Here's how the part is built. I have some questions about the finished solid (model axes, mm). Face numbers are marked on the shaded views. A direction names the side the tool comes from. Round coordinates to 2 decimals unless told otherwise and drop trailing zeros. Loops run counter-clockwise (first coordinate to the right, second up) from the corner with the lowest first, then second, coordinate; pieces in that order, holes last. Notation, with made-up numbers: (44.25, -12.5) -> (58.25, -12.5) arc R18 cw to (58.25, 17.5) -> close; hole circle Ø3 at (21, 34.25). An arc over 180 degrees is marked (long way). One line per item, written item: value. Start each with the question number.
```python
from build123d import *

# Parameters (mm, degrees)
SKETCH_1_R              = 1.75
EXTRUDE_1_DEPTH         = 3.5
EXTRUDE_2_DEPTH         = 1.5
EXTRUDE_2_DEPTH_BACK    = 13.5
SKETCH_2_R              = 5
SKETCH_2_R_2            = 4
CUT_EXTRUDE_START       = -3.5
CUT_EXTRUDE_1_OUTLINE_R = 4
CUT_EXTRUDE_1_DEPTH     = 3.5


# Read off the part's stored shape, not the designer's step: the extrude step
with BuildPart() as part:
    # Sketch 1 → Extrude 1 (new body)
    with BuildSketch(Plane.XY):
        with BuildLine():
            Line((-9.5, -5.5), (9.5, -5.5))
            ThreePointArc((9.5, -5.5), (11, 0), (9.5, 5.5))
            Line((9.5, 5.5), (-9.5, 5.5))
            ThreePointArc((-9.5, 5.5), (-11, 0), (-9.5, -5.5))
        make_face()
        with Locations((8, 0)):
            Circle(SKETCH_1_R, mode=Mode.SUBTRACT)
        with Locations((-8, 0)):
            Circle(SKETCH_1_R, mode=Mode.SUBTRACT)
    extrude(amount=EXTRUDE_1_DEPTH)

    # Sketch 2 → Extrude 2 (add, two sides: drawn at the far end of the back side and taken through both)
    with BuildSketch(Plane(origin=(0, 0, 0), x_dir=(-1, 0, 0), z_dir=(0, 0, -1)).offset(-EXTRUDE_2_DEPTH_BACK)):
        Circle(SKETCH_2_R)
        Circle(SKETCH_2_R_2, mode=Mode.SUBTRACT)
    extrude(amount=EXTRUDE_2_DEPTH + EXTRUDE_2_DEPTH_BACK)

    # Cut-Extrude 1 outline → Cut-Extrude 1 (cut)
    with BuildSketch(Plane(origin=(0, 0, 0), x_dir=(-1, 0, 0), z_dir=(0, 0, -1)).offset(CUT_EXTRUDE_START)):
        Circle(CUT_EXTRUDE_1_OUTLINE_R)
    extrude(amount=CUT_EXTRUDE_1_DEPTH, mode=Mode.SUBTRACT)


solid = part.part
```
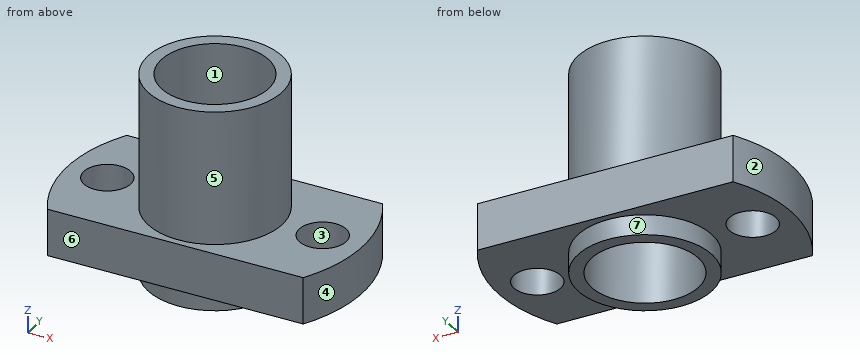
Q1. Which directions (+Z, -Z, +X, -X, +Y, -Y) give clear straight access to the entire face, cutting with the end or side of a thin tool? Please do the marked faces 5, 6 and 7.
Q2. I want a section at B-B on x = -8. Please give me the cut outline in (y, z).
Q3. If we mould it in two halves opening along X, with no side actions, what happens to the marked faces 1, 2, 3 and 4? For each: released by +X, released by -X, zero draft, split by the parting line, or undercut.
Q4. I want a section at A-A on y = 0. Please give me the cut outline in (x, z).
Q5. I want a section at D-D on y = -4.25. Please give me the cut outline in (x, z), plus the area to 3 significant figures.
Q6. Will these pins go through, and if not, where does the flat tip stop? P1, Ø2, axis at y = -3.5, z = 8.5, coming from the +X side; P2, Ø3.5, axis at x = -1.5, y = 2, coming from the -Z side; P3, Ø4, axis at y = -1.5, z = 6, coming from the +X side; P4, Ø2, axis at x = -1, z = 11.5, coming from the -Y side.
Q7. I want a section at C-C on z = 2.75. Please give me the cut outline in (x, y), plus the area to 3 significant figures.
Q8. If I drill on line 1 along Y through (x, z) = (8, 1); line 2 along X through (y, z) = (0.75, 3.25); line 3 along Y through (x, z) = (0, 9), over which ranges is the centre line in solid material (lowest first)?
Answers below:
1. face 5: +Z
1. face 6: +Z, -Z, +X, -X, -Y
1. face 7: -Z
2. outline: (-5.5, 0) -> (-1.75, 0) -> (-1.75, 3.5) -> (-5.5, 3.5) -> close; (1.75, 0) -> (5.5, 0) -> (5.5, 3.5) -> (1.75, 3.5) -> close
3. face 1: undercut
3. face 2: released by -X
3. face 3: undercut
3. face 4: released by +X
4. outline: (-11, 0) -> (-9.75, 0) -> (-9.75, 3.5) -> (-11, 3.5) -> close; (-6.25, 0) -> (-5, 0) -> (-5, -1.5) -> (-4, -1.5) -> (-4, 13.5) -> (-5, 13.5) -> (-5, 3.5) -> (-6.25, 3.5) -> close; (4, -1.5) -> (5, -1.5) -> (5, 0) -> (6.25, 0) -> (6.25, 3.5) -> (5, 3.5) -> (5, 13.5) -> (4, 13.5) -> close; (9.75, 0) -> (11, 0) -> (11, 3.5) -> (9.75, 3.5) -> close
5. outline: (-10.13, 0) -> (-2.63, 0) -> (-2.63, -1.5) -> (2.63, -1.5) -> (2.63, 0) -> (10.13, 0) -> (10.13, 3.5) -> (2.63, 3.5) -> (2.63, 13.5) -> (-2.63, 13.5) -> (-2.63, 3.5) -> (-10.13, 3.5) -> close
5. area: 132 mm^2
6. P1: stops at x = 4.33
6. P2: stops at z = -1.5
6. P3: stops at x = 5
6. P4: stops at y = -5
7. outline: (-9.5, -5.5) -> (9.5, -5.5) arc R10.83 ccw to (9.5, 5.5) -> (-9.5, 5.5) arc R10.83 ccw to start; hole circle Ø3.5 at (-8, 0); hole circle Ø8 at (0, 0); hole circle Ø3.5 at (8, 0)
7. area: 162 mm^2
8. line 1: y = -5.5 to -1.75, 1.75 to 5.5
8. line 2: x = -10.97 to -9.58, -6.42 to -3.93, 3.93 to 6.42, 9.58 to 10.97
8. line 3: y = -5 to -4, 4 to 5
